For this review, use the dimensioned drawing (mm, ordinates from the lowest corner) and the shaded views. Give positions to 0.01 mm unless a question says otherwise; leave off trailing zeros. Write each loop counter-clockwise with the first axis right and the second up, starting at its lowest first coordinate (ties: lowest second). Pieces come first, ordered by that corner, then holes. Notation, with made-up numbers: (62, -10.5) - (81, -10.5) arc R28 cw to (81, 14.5) - close; hole circle Ø7 at (38.25, -35). An arc over 180 degrees is marked (long way). Use a Markdown table: item, result. Add a question column.
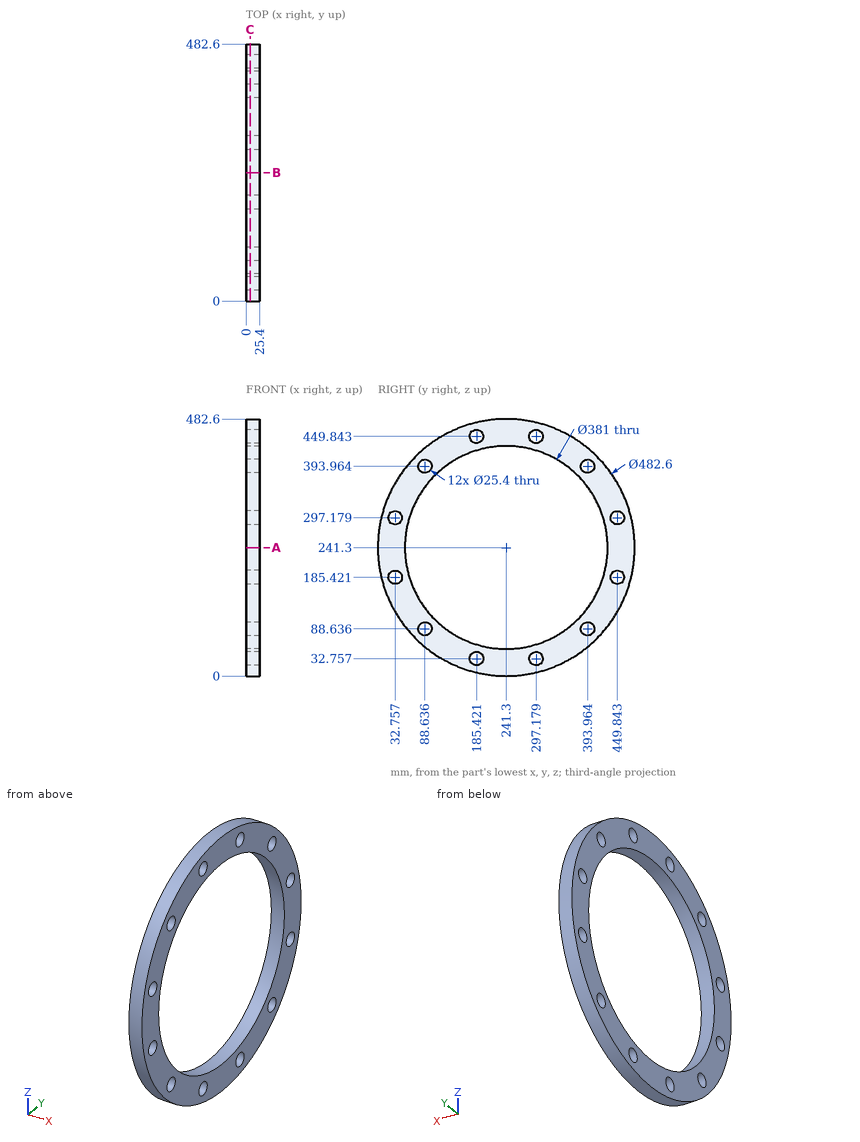
(1) Insertion check: pin 1 (12 mm diameter, centred on x = 6.5, y = 330.5, fed in from -Z); pin 2 (12 mm diameter, centred on x = 7.5, z = 100.5, fed in from -Y); pin 3 (4 mm diameter, centred on x = 15, y = 291.5, fed in from -Z). Each pin has a flat end and moves straight along its axis. Give the tip position at first contact, or say it passes through.
(2) Add section C-C (x = 7.5). Count the separate pieces of the cut face and the enclosed holes in it, and give its area (3 significant figures).
(3) Add section A-A (z = 241.3). State the section outline as (x, y) points, and give its area (3 significant figures).
(4) For line 1 along Z through (x, y) = (2.75, 247) (1 decimal); line 2 along Y through (x, z) = (21.25, 386) (1 decimal); line 3 along Y through (x, z) = (12, 241.3), list the stretches that pass through material, from the lowest coordinate up.
Answers follow:
| question | item | result |
|---|---|---|
| 1 | pin 1 | z = 14.8 |
| 1 | pin 2 | y = 41.16 |
| 1 | pin 3 | z = 4.86 |
| 2 | separate pieces | 1 |
| 2 | enclosed holes | 13 |
| 2 | area | 62,800 mm^2 |
| 3 | outline | (0, 0) - (25.4, 0) - (25.4, 50.8) - (0, 50.8) - close; (0, 431.8) - (25.4, 431.8) - (25.4, 482.6) - (0, 482.6) - close |
| 3 | area | 2,580 mm^2 |
| 4 | line 1 | 0.1 to 50.9, 431.7 to 482.5 |
| 4 | line 2 | 48.2 to 78.7, 98.5 to 117.4, 365.2 to 384.1, 403.9 to 434.4 |
| 4 | line 3 | 0 to 50.8, 431.8 to 482.6 |
